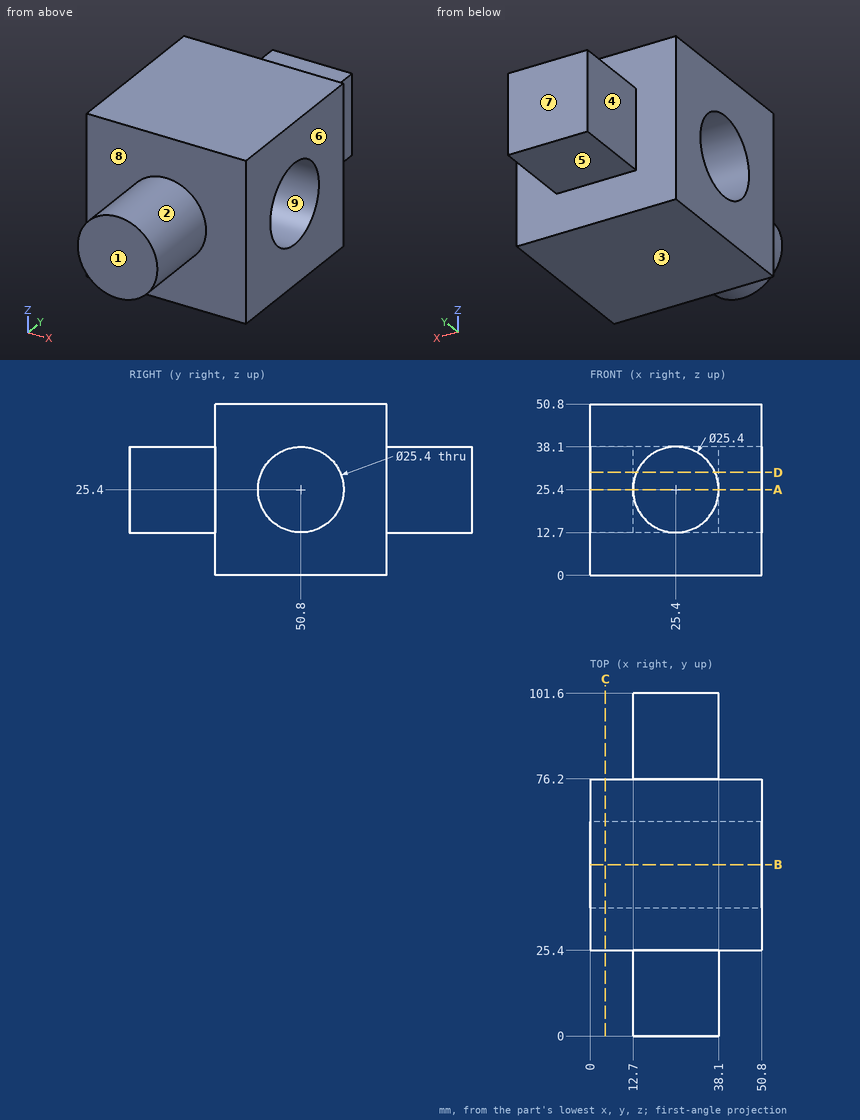
The drawing under review shows one solid part. Ordinate dimensions are in mm from its lowest x, y, z. A direction names the side the tool comes from. Round coordinates to 2 decimals unless told otherwise and drop trailing zeros. Loops run counter-clockwise (first coordinate to the right, second up) from the corner with the lowest first, then second, coordinate; pieces in that order, holes last. Notation, with made-up numbers: (17.25, 1.5) - (35.25, 1.5) arc R5 cw to (35.25, 6.5) - close; hole circle Ø11 at (35.25, -35). An arc over 180 degrees is marked (long way). One line per item, written item: value. Start each with the question number.
1) Draft analysis for pull direction Y (two halves, no side actions). For the marked faces 6, 7, 8 and 9, state which applies: +Y half, -Y half, draft (parallel to the pull), parting line (faces both ways), or undercut.
2) Insertion check: pin 1 Ø20.5 at (y, z) = (93, 24) entering from +X; pin 2 Ø7.5 at (x, y) = (20.5, 84.5) entering from +Z; pin 3 Ø12.5 at (y, z) = (91.5, 20) entering from -X. Each pin has a flat end and moves straight along its axis. Give the tip position at first contact, or say it passes through.
3) Consider section B-B on y = 50.8. Give the boundary of the cut face in (x, z).
4) For the marked faces 1, 2, 3, 4 and 5, list the 3-axis set-ups (+Z, -Z, +X, -X, +Y, -Y) from which the entire face can be reached by the end or side of a thin tool; tool diameter is ignored.
5) Consider section D-D on z = 30.5. Give the boundary of the cut face in (x, y).
6) Consider section A-A on z = 25.4. Give the boundary of the cut face in (x, y), then the cut area to 3 significant figures.
7) Consider section C-C on x = 4.5. Give the boundary of the cut face in (y, z), then the cut area to 3 significant figures.
8) To check wall thickness, follow L1, parallel to Z at x = 32, y = 50.8; L2, parallel to Y at x = 9, z = 25.5; L3, parallel to Z at x = 5, y = 62. State the ranges of each line that lie inside material, in increasing order. Write a range as from..to.
Reported:
1. face 6: draft
1. face 7: +Y half
1. face 8: -Y half
1. face 9: undercut
2. pin 1: stops at x = 38.1
2. pin 2: stops at z = 38.1
2. pin 3: stops at x = 12.7
3. outline: (0, 0) - (50.8, 0) - (50.8, 12.7) - (0, 12.7) - close; (0, 38.1) - (50.8, 38.1) - (50.8, 50.8) - (0, 50.8) - close
4. face 1: +Z, -Z, +X, -X, -Y
4. face 2: -Y
4. face 3: -Z, +X, -X, +Y, -Y
4. face 4: +Z, -Z, -X, +Y
4. face 5: -Z, +X, -X, +Y
5. outline: (0, 25.4) - (13.77, 25.4) - (13.77, 0) - (37.03, 0) - (37.03, 25.4) - (50.8, 25.4) - (50.8, 39.17) - (0, 39.17) - close; (0, 62.43) - (50.8, 62.43) - (50.8, 76.2) - (38.1, 76.2) - (38.1, 101.6) - (12.7, 101.6) - (12.7, 76.2) - (0, 76.2) - close
6. outline: (0, 25.4) - (12.7, 25.4) - (12.7, 0) - (38.1, 0) - (38.1, 25.4) - (50.8, 25.4) - (50.8, 38.1) - (0, 38.1) - close; (0, 63.5) - (50.8, 63.5) - (50.8, 76.2) - (38.1, 76.2) - (38.1, 101.6) - (12.7, 101.6) - (12.7, 76.2) - (0, 76.2) - close
6. area: 2,580 mm^2
7. outline: (25.4, 0) - (76.2, 0) - (76.2, 50.8) - (25.4, 50.8) - close; hole circle Ø25.4 at (50.8, 25.4)
7. area: 2,070 mm^2
8. L1: z = 0..12.7, 38.1..50.8
8. L2: y = 25.4..38.1, 63.5..76.2
8. L3: z = 0..19.41, 31.39..50.8
